```python
from build123d import *

# Parameters (mm, degrees)
SKETCH2_W                 = 75.4
SKETCH2_H                 = 50
BOSS_EXTRUDE1_DEPTH       = 3.5
SKETCH3_R                 = 1.5
CUT_EXTRUDE1_DEPTH        = 4
BOSS_EXTRUDE2_START       = 8
SKETCH4_R                 = 3
SKETCH4_R_2               = 1.5
BOSS_EXTRUDE2_DEPTH       = 8
MIRROR2_START             = 8
MIRROR2_COPY_1_SKETCH_R   = 3
MIRROR2_COPY_1_SKETCH_R_2 = 1.5
MIRROR2_COPY_1_DEPTH      = 8
FILLET1_R                 = 2
SKETCH6_W                 = 75.4
SKETCH6_H                 = 50
BOSS_EXTRUDE3_DEPTH       = 4
SKETCH9_R                 = 8.55
CUT_EXTRUDE2_DEPTH        = 1.5
SKETCH10_R                = 4.85
CUT_EXTRUDE3_DEPTH        = 1.87
SKETCH11_R                = 4
CUT_EXTRUDE4_DEPTH        = 0.5
CUT_EXTRUDE6_DEPTH        = 1.87
SKETCH14_W                = 8
SKETCH14_H                = 6
BOSS_EXTRUDE6_DEPTH       = 8
SKETCH15_R                = 1.6
CUT_EXTRUDE7_DEPTH        = 8
SKETCH16_W                = 4
SKETCH16_H                = 5
CUT_EXTRUDE8_DEPTH        = 8
SKETCH17_W                = 8
SKETCH17_H                = 6
CUT_EXTRUDE9_DEPTH        = 1


with BuildPart() as part:
    # Sketch2 → Boss-Extrude1 (new body)
    with BuildSketch(Plane(origin=(0, 0, 0), x_dir=(1, 0, 0), z_dir=(0, 1, 0))):
        with Locations((37.7, 25)):
            Rectangle(SKETCH2_W, SKETCH2_H)
    extrude(amount=BOSS_EXTRUDE1_DEPTH)

    # Sketch3 → Cut-Extrude1 (cut)
    with BuildSketch(Plane(origin=(0, 3.5, 0), x_dir=(1, 0, 0), z_dir=(0, 1, 0))):
        with Locations(Location((12.3, 37.7, 0), (0, 0, 270))):
            Circle(SKETCH3_R)
        with Locations(Location((12.3, 12.3, 0), (0, 0, 270))):
            Circle(SKETCH3_R)
        with Locations(Location((63.1, 37.7, 0), (0, 0, 270))):
            Circle(SKETCH3_R)
        with Locations(Location((63.1, 12.3, 0), (0, 0, 270))):
            Circle(SKETCH3_R)
    extrude(amount=-CUT_EXTRUDE1_DEPTH, mode=Mode.SUBTRACT)

    # Sketch4 → Boss-Extrude2 (add)
    with BuildSketch(Plane(origin=(0, 3.5, 0), x_dir=(1, 0, 0), z_dir=(0, 1, 0)).offset(BOSS_EXTRUDE2_START)):
        with Locations(Location((12.3, 37.7, 0), (0, 0, 90))):
            Circle(SKETCH4_R)
        with Locations(Location((12.3, 37.7, 0), (0, 0, 270))):
            Circle(SKETCH4_R_2, mode=Mode.SUBTRACT)
    boss_extrude2 = extrude(amount=-BOSS_EXTRUDE2_DEPTH)

    # Mirror1: Boss-Extrude2 across plane
    add(boss_extrude2.mirror(Plane.XY.offset(-25)))

    # Mirror2: Boss-Extrude2 across plane
    add(boss_extrude2.mirror(Plane.ZY.offset(-37.7)))

    # Mirror2 copy 1 sketch → Mirror2 copy 1 (add)
    with BuildSketch(Plane(origin=(75.4, 3.5, -50), x_dir=(-1, 0, 0), z_dir=(0, 1, 0)).offset(MIRROR2_START)):
        with Locations(Location((12.3, 37.7, 0), (0, 0, 90))):
            Circle(MIRROR2_COPY_1_SKETCH_R)
        with Locations(Location((12.3, 37.7, 0), (0, 0, 270))):
            Circle(MIRROR2_COPY_1_SKETCH_R_2, mode=Mode.SUBTRACT)
    extrude(amount=-MIRROR2_COPY_1_DEPTH)

    # Fillet1
    fillet1_edges = [part.edges().sort_by_distance(p)[0] for p in [
        (12.3, 3.5, -34.7),
        (12.3, 3.5, -15.3),
        (63.1, 3.5, -15.3),
        (63.1, 3.5, -34.7),
    ]]
    fillet(fillet1_edges, radius=FILLET1_R)

    # Sketch6 → Boss-Extrude3 (add)
    with BuildSketch(Plane.XZ):
        with Locations((37.7, -25)):
            Rectangle(SKETCH6_W, SKETCH6_H)
    extrude(amount=-BOSS_EXTRUDE3_DEPTH)

    # Sketch9 → Cut-Extrude2 (cut)
    with BuildSketch(Plane(origin=(0, 4, 0), x_dir=(1, 0, 0), z_dir=(0, 1, 0))):
        with Locations(Location((37.7, 25, 0), (0, 0, 270))):
            Circle(SKETCH9_R)
    extrude(amount=-CUT_EXTRUDE2_DEPTH, mode=Mode.SUBTRACT)

    # Sketch10 → Cut-Extrude3 (cut)
    with BuildSketch(Plane.XZ):
        with Locations(Location((17.699747997, -25, 0), (0, 0, 270))):
            Circle(SKETCH10_R)
    extrude(amount=-CUT_EXTRUDE3_DEPTH, mode=Mode.SUBTRACT)

    # Sketch11 → Cut-Extrude4 (cut)
    with BuildSketch(Plane.XZ.offset(-1.87)):
        with Locations(Location((17.699747997, -25, 0), (0, 0, 270))):
            Circle(SKETCH11_R)
    extrude(amount=-CUT_EXTRUDE4_DEPTH, mode=Mode.SUBTRACT)

    # Sketch12 → Cut-Extrude6 (cut)
    with BuildSketch(Plane.XZ):
        with BuildLine():
            Line((12.849747997, -25), (12.849747997, -27.5))
            Line((12.849747997, -27.5), (13.543728267, -27.5))
            ThreePointArc((13.543728267, -27.5), (13.026462445, -26.297267187), (12.849747997, -25))
        make_face()
        with BuildLine():
            Line((12.849747997, -22.5), (12.849747997, -25))
            ThreePointArc((12.849747997, -25), (13.026462445, -23.702732813), (13.543728267, -22.5))
            Line((13.543728267, -22.5), (12.849747997, -22.5))
        make_face()
        Polygon((0, -22.5), (0, -27.5), (12.849747997, -27.5), (12.849747997, -25), (12.849747997, -22.5), align=None)
    extrude(amount=-CUT_EXTRUDE6_DEPTH, mode=Mode.SUBTRACT)

    # Sketch14 → Boss-Extrude6 (add)
    with BuildSketch(Plane.XZ):
        with Locations((67.4, -7)):
            Rectangle(SKETCH14_W, SKETCH14_H)
    boss_extrude6 = extrude(amount=BOSS_EXTRUDE6_DEPTH)

    # Sketch15 → Cut-Extrude7 (cut)
    with BuildSketch(Plane(origin=(0, 0, -10), x_dir=(-1, 0, 0), z_dir=(0, 0, -1))):
        with Locations((-67.4, -4)):
            Circle(SKETCH15_R)
    cut_extrude7 = extrude(amount=-CUT_EXTRUDE7_DEPTH, mode=Mode.SUBTRACT)

    # Mirror4: Boss-Extrude6, Cut-Extrude7 across plane
    add(boss_extrude6.mirror(Plane.XY.offset(-25)))
    add(cut_extrude7.mirror(Plane.XY.offset(-25)), mode=Mode.SUBTRACT)

    # Sketch16 → Cut-Extrude8 (cut)
    with BuildSketch(Plane.XZ):
        Polygon((4, -46), (4, -27.5), (0, -27.5), (0, -50), (4, -50), align=None)
        with Locations((2, -25)):
            Rectangle(SKETCH16_W, SKETCH16_H)
        Polygon((4, -22.5), (4, -4), (4, 0), (0, 0), (0, -22.5), align=None)
        Polygon((63.4, -4), (71.4, -4), (71.4, -10), (71.4, -40), (71.4, -46), (63.4, -46), (4, -46), (4, -50), (75.4, -50), (75.4, 0), (4, 0), (4, -4), align=None)
    extrude(amount=-CUT_EXTRUDE8_DEPTH, mode=Mode.SUBTRACT)

    # Sketch17 → Cut-Extrude9 (cut)
    with BuildSketch(Plane.XZ.offset(8)):
        with Locations((67.4, -43)):
            Rectangle(SKETCH17_W, SKETCH17_H)
        with Locations((67.4, -7)):
            Rectangle(SKETCH17_W, SKETCH17_H)
    extrude(amount=-CUT_EXTRUDE9_DEPTH, mode=Mode.SUBTRACT)


solid = part.part
```
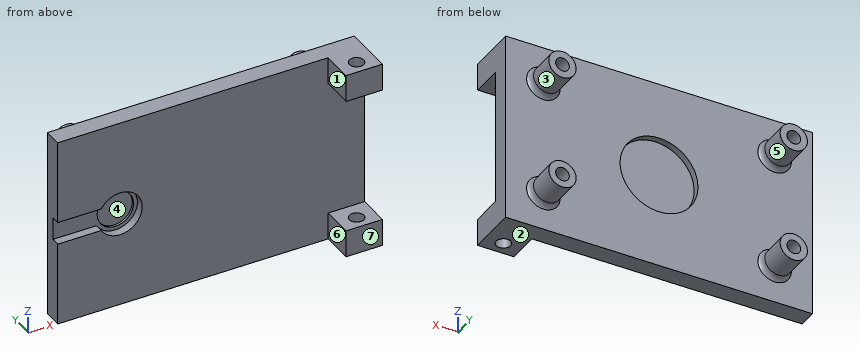
The model under review builds one solid part; all positions refer to its coordinate system, in mm. Face numbers are marked on the shaded views. A direction names the side the tool comes from. Coordinates: 2 decimals unless noted, no trailing zeros. Loops run counter-clockwise (first coordinate to the right, second up) from the corner with the lowest first, then second, coordinate; pieces in that order, holes last. Notation, with made-up numbers: (64.5, 35.25) -> (103.5, 35.25) arc R34 ccw to (103.5, 71.25) -> close; hole circle Ø8 at (30.25, -18). An arc over 180 degrees is marked (long way). Answer as CSV lines item,"result".
Item 1: Take a section at C-C, the plane x = 37.7. State the section outline as (y, z) points.
Results below:
outline,"(0, -46) -> (4, -46) -> (4, -33.55) -> (2.5, -33.55) -> (2.5, -16.45) -> (4, -16.45) -> (4, -4) -> (0, -4) -> close"
Item 2: Take a section at D-D, the plane z = -25. State the section outline as (x, y) points, and give its area (3 significant figures).
Results below:
outline,"(4, 1.87) -> (13.7, 1.87) -> (13.7, 2.37) -> (21.7, 2.37) -> (21.7, 1.87) -> (22.55, 1.87) -> (22.55, 0) -> (71.4, 0) -> (71.4, 4) -> (46.25, 4) -> (46.25, 2.5) -> (29.15, 2.5) -> (29.15, 4) -> (4, 4) -> close"
area,"205 mm2"
Item 3: For L1, parallel to X at y = 6.25, z = -37.7; L2, parallel to Y at x = 33.5, z = -41; L3, parallel to X at y = -4, z = -42.75, list the stretches that pass through material, from the lowest coordinate up.
Results below:
L1,"x = 9.3 to 10.8, 13.8 to 15.3, 60.1 to 61.6, 64.6 to 66.1"
L2,"y = 0 to 4"
L3,"x = 63.4 to 65.8, 69 to 71.4"
Item 4: Take a section at B-B, the plane y = -4. State the section outline as (x, z) points, and give its area (3 significant figures).
Results below:
outline,"(63.4, -46) -> (65.8, -46) -> (65.8, -40) -> (63.4, -40) -> close; (63.4, -10) -> (65.8, -10) -> (65.8, -4) -> (63.4, -4) -> close; (69, -46) -> (71.4, -46) -> (71.4, -40) -> (69, -40) -> close; (69, -10) -> (71.4, -10) -> (71.4, -4) -> (69, -4) -> close"
area,"57.6 mm2"
Item 5: Draft analysis for pull direction X (two halves, no side actions). For the marked faces 5, 6 and 7, state which applies: +X half, -X half, draft (parallel to the pull), parting line (faces both ways), or undercut.
Results below:
face 5,"undercut"
face 6,"-X half"
face 7,"draft"
Item 6: Machinability: for the marked faces 1, 2, 3 and 4, which of the approach directions +Z, -Z, +X, -X, +Y, -Y give a long, thin tool a straight path to every point of the face, cutting with its end or side? Answer none if there is none.
Results below:
face 1,"+Z, -Z, -X, -Y"
face 2,"-Z, +X, -X, +Y, -Y"
face 3,"+Y"
face 4,"-Y"
Item 7: Insertion check: pin 1 (1.5 mm diameter, centred on x = 63.5, z = -12, fed in from +Y); pin 2 (3 mm diameter, centred on y = -5, z = -42.5, fed in from -X); pin 3 (12.5 mm diameter, centred on x = 17.7, z = -25, fed in from -Y). Each pin has a flat end and moves straight along its axis. Give the tip position at first contact, or say it passes through.
Results below:
pin 1,"stops at y = 4"
pin 2,"stops at x = 63.4"
pin 3,"stops at y = 0"
Item 8: Take a section at A-A, the plane y = 10. State the section outline as (x, z) points, and give its area (3 significant figures).
Results below:
outline,"circle Ø6 at (12.3, -37.7); circle Ø6 at (12.3, -12.3); circle Ø6 at (63.1, -37.7); circle Ø6 at (63.1, -12.3); hole circle Ø3 at (12.3, -37.7); hole circle Ø3 at (12.3, -12.3); hole circle Ø3 at (63.1, -37.7); hole circle Ø3 at (63.1, -12.3)"
area,"84.8 mm2"
